Build history of the part. All positions in model axes, mm. Give positions to 0.01 mm unless a question says otherwise; leave off trailing zeros. Order: outer loops, then holes, each group sorted by start corner. A loop starts at its lowest first (then second) coordinate and runs counter-clockwise, first axis right, second up. Notation, with made-up numbers: M 34.25,22 L 60.25,22 A21 cw 60.25,38 Z; hole C -9.75,-2 d6. An arc over 180 degrees is marked long. Use CSV: the item, a comma, the result in double quotes. Start each with the question number.
Item 1: Band-saw the part on B-B on x = 31. Write the cut outline in (y, z).
Item 2: Band-saw the part on C-C on z = -40. Write the cut outline in (x, y), plus the area to 3 significant figures.
Item 3: Pin check, flat tips, straight feed: P1, Ø0.8, axis at y = 1.5, z = -33, coming from the -X side; P2, Ø3.5, axis at x = -128.88, z = 2.73, coming from the +Y side; P3, Ø0.9, axis at x = -160.5, y = 2, coming from the -Z side. Stop position of each tip, or through.
Item 4: Band-saw the part on A-A on y = 0.5. Write the cut outline in (x, z), plus the area to 3 significant figures.
Item 5: Wall check: line 1 along X through (y, z) = (2.65, -33); line 2 along Z through (x, y) = (32, 0.9); line 3 along Z through (x, y) = (78.5, 0.6). Give the ranges that are in metal, low to high.
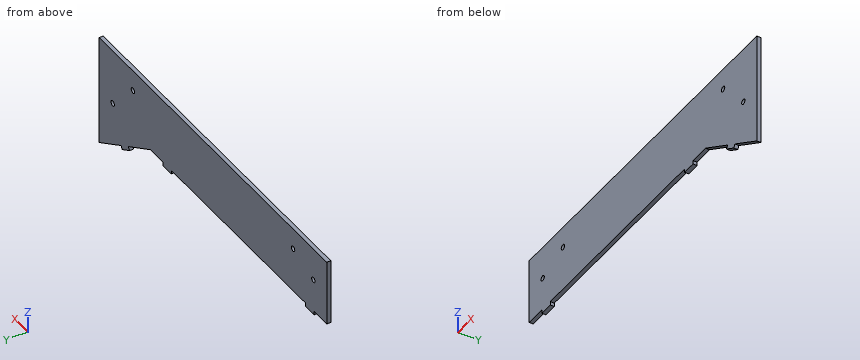
from build123d import *

# Parameters (mm, degrees)
BOSS_EXTRUDE1_DEPTH = 3
CUT_EXTRUDE1_REACH  = 5
SKETCH2_R           = 2
CUT_EXTRUDE2_REACH  = 5
SKETCH3_R           = 2
SKETCH4_W           = 10
SKETCH4_H           = 3
BOSS_EXTRUDE3_DEPTH = 2.7
SKETCH5_W           = 10
SKETCH5_H           = 3
BOSS_EXTRUDE4_DEPTH = 2.7


with BuildPart() as part:
    # Sketch1 → Boss-Extrude1 (new body)
    with BuildSketch(Plane(origin=(0, 0, 0), x_dir=(1, 0, 0), z_dir=(0, 1, 0))):
        Polygon((101.124303582, 11.213732055), (101.124303582, 66.273277114), (40.502525317, 31.273277114), (-168.875696418, 31.273277114), (-168.875696418, -18.726722886), (101.124303582, -18.726722886), align=None)
    extrude(amount=BOSS_EXTRUDE1_DEPTH)

    # Sketch2 → Cut-Extrude1 (cut, up to next)
    with BuildSketch(Plane(origin=(0, 3, 0), x_dir=(1, 0, 0), z_dir=(0, 1, 0)), mode=Mode.PRIVATE) as cut_extrude1_sk1:
        with Locations(Location((-152.875696418, 6.273277114, 0), (0, 0, 270))):  # turned: the seam where the file's is
            Circle(SKETCH2_R)
    cut_extrude1_tool1 = extrude(cut_extrude1_sk1.sketch, amount=-CUT_EXTRUDE1_REACH, mode=Mode.PRIVATE) & part.part
    add(cut_extrude1_tool1.solids().sort_by_distance((-152.875696, 3, -6.273277))[0], mode=Mode.SUBTRACT)
    # Sketch2 → Cut-Extrude1 (cut, up to next)
    with BuildSketch(Plane(origin=(0, 3, 0), x_dir=(1, 0, 0), z_dir=(0, 1, 0)), mode=Mode.PRIVATE) as cut_extrude1_sk2:
        with Locations(Location((85.124303582, 23.773277114, 0), (0, 0, 270))):  # turned: the seam where the file's is
            Circle(SKETCH2_R)
    cut_extrude1_tool2 = extrude(cut_extrude1_sk2.sketch, amount=-CUT_EXTRUDE1_REACH, mode=Mode.PRIVATE) & part.part
    add(cut_extrude1_tool2.solids().sort_by_distance((85.124304, 3, -23.773277))[0], mode=Mode.SUBTRACT)

    # Sketch3 → Cut-Extrude2 (cut, up to next)
    with BuildSketch(Plane(origin=(0, 3, 0), x_dir=(1, 0, 0), z_dir=(0, 1, 0)), mode=Mode.PRIVATE) as cut_extrude2_sk1:
        with Locations(Location((-128.875696418, -2.726722886, 0), (0, 0, 270))):  # turned: the seam where the file's is
            Circle(SKETCH3_R)
    cut_extrude2_tool1 = extrude(cut_extrude2_sk1.sketch, amount=-CUT_EXTRUDE2_REACH, mode=Mode.PRIVATE) & part.part
    add(cut_extrude2_tool1.solids().sort_by_distance((-128.875696, 3, 2.726723))[0], mode=Mode.SUBTRACT)
    # Sketch3 → Cut-Extrude2 (cut, up to next)
    with BuildSketch(Plane(origin=(0, 3, 0), x_dir=(1, 0, 0), z_dir=(0, 1, 0)), mode=Mode.PRIVATE) as cut_extrude2_sk2:
        with Locations(Location((61.124303582, -2.726722886, 0), (0, 0, 270))):  # turned: the seam where the file's is
            Circle(SKETCH3_R)
    cut_extrude2_tool2 = extrude(cut_extrude2_sk2.sketch, amount=-CUT_EXTRUDE2_REACH, mode=Mode.PRIVATE) & part.part
    add(cut_extrude2_tool2.solids().sort_by_distance((61.124304, 3, 2.726723))[0], mode=Mode.SUBTRACT)

    # Sketch4 → Boss-Extrude3 (add)
    with BuildSketch(Plane.XY.offset(-31.273277114)):
        with Locations((-148.875696418, 1.5)):
            Rectangle(SKETCH4_W, SKETCH4_H)
        with Locations((20.502525317, 1.5)):
            Rectangle(SKETCH4_W, SKETCH4_H)
    extrude(amount=-BOSS_EXTRUDE3_DEPTH)

    # Sketch5 → Boss-Extrude4 (add)
    with BuildSketch(Plane(origin=(-3.416094891, 0, -5.916849915), x_dir=(-0.866025404, 0, 0.5), z_dir=(-0.5, 0, -0.866025404))):
        with Locations((-85.712854399, 1.5)):
            Rectangle(SKETCH5_W, SKETCH5_H)
    extrude(amount=BOSS_EXTRUDE4_DEPTH)


solid = part.part
Model answer:
1,outline,"M 0,-31.27 L 3,-31.27 L 3,18.73 L 0,18.73 Z"
2,outline,"M 55.62,0 L 101.12,0 L 101.12,3 L 55.62,3 Z"
2,area,"137 mm^2"
3,P1,"stops at x = -153.88"
3,P2,"passes through"
3,P3,"stops at z = -31.27"
4,outline,"M -168.88,-31.27 L -153.88,-31.27 L -153.88,-33.97 L -143.88,-33.97 L -143.88,-31.27 L 15.5,-31.27 L 15.5,-33.97 L 25.5,-33.97 L 25.5,-31.27 L 40.5,-31.27 L 66.48,-46.27 L 65.13,-48.61 L 73.79,-53.61 L 75.14,-51.27 L 101.12,-66.27 L 101.12,18.73 L -168.88,18.73 Z; hole C -152.88,-6.27 d4; hole C -128.88,2.73 d4; hole C 61.12,2.73 d4; hole C 85.12,-23.77 d4"
4,area,"14,600 mm^2"
5,line 1,"x = -153.88 to -143.88, 15.5 to 25.5, 43.49 to 101.12"
5,line 2,"z = -31.27 to 18.73"
5,line 3,"z = -53.21 to 18.73"
